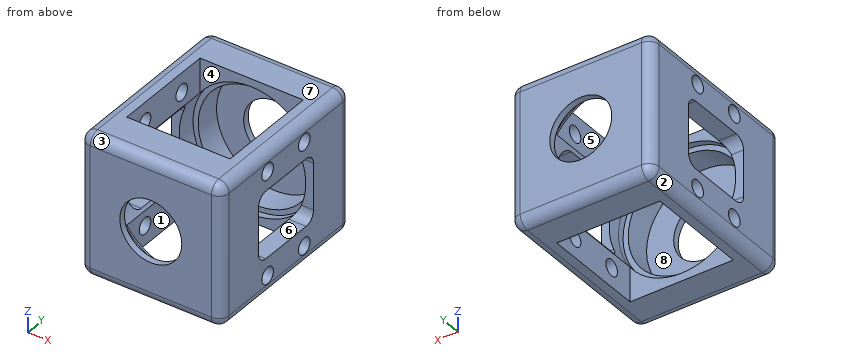
from build123d import *

# Parameters (mm, degrees)
SKETCH1_W               = 34.925
SKETCH1_H               = 34.925
SKETCH1_R               = 7.62
BOSS_EXTRUDE1_DEPTH     = 44.45
SKETCH2_W               = 25.4
SKETCH2_H               = 25.4
CUT_EXTRUDE1_DEPTH      = 44.45
SKETCH3_R               = 15.5575
CUT_EXTRUDE2_DEPTH      = 27.0002
CUT_EXTRUDE2_DEPTH_BACK = 1.6002
SKETCH4_R               = 14.2875
CUT_EXTRUDE3_DEPTH      = 34.9504
CUT_EXTRUDE3_DEPTH_BACK = 6.35
SKETCH5_W               = 16.51
SKETCH5_H               = 19.05
CUT_EXTRUDE4_DEPTH      = 228.6
SKETCH6_R               = 2
CUT_EXTRUDE5_DEPTH      = 228.6
FILLET1_R               = 2.54


with BuildPart() as part:
    # Sketch1 → Boss-Extrude1 (new body)
    with BuildSketch(Plane(origin=(0, 0, 0), x_dir=(1, 0, 0), z_dir=(0, 1, 0))):
        Rectangle(SKETCH1_W, SKETCH1_H)
        Circle(SKETCH1_R, mode=Mode.SUBTRACT)
    extrude(amount=BOSS_EXTRUDE1_DEPTH)

    # Sketch2 → Cut-Extrude1 (cut)
    with BuildSketch(Plane.XY.offset(17.4625)):
        with Locations((0, 22.225)):
            Rectangle(SKETCH2_W, SKETCH2_H)
    extrude(amount=-CUT_EXTRUDE1_DEPTH, mode=Mode.SUBTRACT)

    # Sketch3 → Cut-Extrude2 (cut, two sides)
    with BuildSketch(Plane(origin=(0, 9.525, 0), x_dir=(1, 0, 0), z_dir=(0, 1, 0))) as cut_extrude2_sk:
        Circle(SKETCH3_R)
    extrude(amount=CUT_EXTRUDE2_DEPTH, mode=Mode.SUBTRACT)
    extrude(cut_extrude2_sk.sketch, amount=-CUT_EXTRUDE2_DEPTH_BACK, mode=Mode.SUBTRACT)

    # Sketch4 → Cut-Extrude3 (cut, two sides)
    with BuildSketch(Plane(origin=(0, 7.9248, 0), x_dir=(1, 0, 0), z_dir=(0, 1, 0))) as cut_extrude3_sk:
        Circle(SKETCH4_R)
    extrude(amount=CUT_EXTRUDE3_DEPTH, mode=Mode.SUBTRACT)
    extrude(cut_extrude3_sk.sketch, amount=-CUT_EXTRUDE3_DEPTH_BACK, mode=Mode.SUBTRACT)

    # Sketch5 → Cut-Extrude4 (cut)
    with BuildSketch(Plane.ZY.offset(17.4625)):
        with Locations((0, 22.225)):
            Rectangle(SKETCH5_W, SKETCH5_H)
    extrude(amount=-CUT_EXTRUDE4_DEPTH, mode=Mode.SUBTRACT)

    # Sketch6 → Cut-Extrude5 (cut)
    with BuildSketch(Plane.ZY.offset(17.4625)):
        with Locations((-12.7, 28.575)):
            Circle(SKETCH6_R)
        with Locations((-12.7, 15.875)):
            Circle(SKETCH6_R)
        with Locations((12.7, 15.875)):
            Circle(SKETCH6_R)
        with Locations((12.7, 28.575)):
            Circle(SKETCH6_R)
    extrude(amount=-CUT_EXTRUDE5_DEPTH, mode=Mode.SUBTRACT)

    # Fillet1
    fillet1_edges = [part.edges().sort_by_distance(p)[0] for p in [
        (-17.4625, 44.45, 0),
        (0, 44.45, 17.4625),
        (17.4625, 44.45, 0),
        (0, 0, 17.4625),
        (-17.4625, 0, 0),
        (0, 0, -17.4625),
        (17.4625, 0, 0),
        (15.324632691, 31.75, 8.255),
        (-15.324632691, 31.75, 8.255),
        (15.324632691, 12.7, 8.255),
        (17.4625, 22.225, 17.4625),
        (15.324632691, 12.7, -8.255),
        (15.324632691, 31.75, -8.255),
        (-17.4625, 22.225, 17.4625),
        (-17.4625, 22.225, -17.4625),
        (-15.324632691, 12.7, 8.255),
        (-15.324632691, 12.7, -8.255),
        (-15.324632691, 31.75, -8.255),
        (17.4625, 22.225, -17.4625),
        (0, 44.45, -17.4625),
    ]]
    fillet(fillet1_edges, radius=FILLET1_R)


solid = part.part
Geometry: final body of the model. Coordinates: model frame, mm. Face numbers are marked on the shaded views. A direction names the side the tool comes from. Round coordinates to 2 decimals unless told otherwise and drop trailing zeros. Order: outer loops, then holes, each group sorted by start corner. A loop starts at its lowest first (then second) coordinate and runs counter-clockwise, first axis right, second up. Notation, with made-up numbers: (32, 12.5) -> (55, 12.5) arc R8 cw to (55, 23.5) -> close; hole circle Ø7 at (57, -39). An arc over 180 degrees is marked (long way). Put each result on its own line as item: value. Start each with the question number.
Q1. Section A-A on y = 38. Return the cut outline in (x, z) (1 decimal), and give its area (3 significant figures).
Q2. Pull-direction query (X, two-part tool) for the marked faces 1, 2, 3 and 4; classes: +X half, -X half, draft (parallel to the pull), parting line (faces both ways), or undercut.
Q3. Section C-C on y = 24.5. Return the cut outline in (x, z) (1 decimal), and give its area (3 significant figures).
Q4. Line query: probe 1 along Y at (x, z) = (15.1, 12.7) (3 decimals); probe 2 along Y at (x, z) = (-10, 12) (3 decimals); probe 3 along Y at (x, z) = (4, 15). Output: solid intervals per line, ascending.
Q5. Section D-D on x = 0. Give the number of separate pieces and of enclosed holes in the cut face, and give its area (3 significant figures).
Q6. Reachability of the marked faces 5, 6, 7 and 8 from +Z, -Z, +X, -X, +Y, -Y: full face, straight path, thin tool, end or side. Return the list, or none.
Ans:
1. outline: (-17.5, -14.9) arc R2.5 ccw to (-14.9, -17.5) -> (14.9, -17.5) arc R2.5 ccw to (17.5, -14.9) -> (17.5, 14.9) arc R2.5 ccw to (14.9, 17.5) -> (-14.9, 17.5) arc R2.5 ccw to (-17.5, 14.9) -> close; hole circle Ø28.6 at (0, 0)
1. area: 573 mm2
2. face 1: undercut
2. face 2: -X half
2. face 3: draft
2. face 4: undercut
3. outline: (-17.5, -14.9) arc R2.5 ccw to (-14.9, -17.5) -> (-12.7, -17.5) -> (-12.7, -9) arc R15.6 cw to (-13.2, -8.3) -> (-17.5, -8.3) -> close; (-17.5, 8.3) -> (-13.2, 8.3) arc R15.6 cw to (-12.7, 9) -> (-12.7, 17.5) -> (-14.9, 17.5) arc R2.5 ccw to (-17.5, 14.9) -> close; (12.7, -17.5) -> (14.9, -17.5) arc R2.5 ccw to (17.5, -14.9) -> (17.5, -8.3) -> (13.2, -8.3) arc R15.6 cw to (12.7, -9) -> close; (12.7, 9) arc R15.6 cw to (13.2, 8.3) -> (17.5, 8.3) -> (17.5, 14.9) arc R2.5 ccw to (14.9, 17.5) -> (12.7, 17.5) -> close
3. area: 169 mm2
4. probe 1: y = 0.006 to 13.875, 17.875 to 26.575, 30.575 to 44.444
4. probe 2: y = 0 to 9.525, 34.925 to 44.45
4. probe 3: y = 0 to 7.92, 36.53 to 44.45
5. separate pieces: 4
5. enclosed holes: 0
5. area: 149 mm2
6. face 5: +Z, -Z
6. face 6: +X, -X
6. face 7: +Z, +X, -X, +Y, -Y
6. face 8: none
